Read the model definition and answer for the solid it produces. Units are mm, in the model's axes. A direction names the side the tool comes from. Give positions to 0.01 mm unless a question says otherwise; leave off trailing zeros. Loops run counter-clockwise (first coordinate to the right, second up) from the corner with the lowest first, then second, coordinate; pieces in that order, holes last. Notation, with made-up numbers: (73.25, -5) - (108.25, -5) arc R15 cw to (108.25, 23) - close; hole circle Ø9 at (88.25, 60). An arc over 180 degrees is marked (long way). Write each question's results on one line, items separated by ' | '. Start each with the question number.
Q1. Given pin 1 (2 mm diameter, centred on x = 74, z = -54, fed in from -Y); pin 2 (12 mm diameter, centred on x = 26.5, z = 53, fed in from +Y); pin 3 (6 mm diameter, centred on x = 40.5, y = -30.5, fed in from -Z) (3 decimals); pin 4 (11.5 mm diameter, centred on x = 39.4, y = 76.21, fed in from -Z) (3 decimals), each flat-ended and moving along its own axis, determine where each tip first touches the part or whether it passes through.
Q2. The part is cut by section B-B, the plane y = 39. Write down the section's boundary in (x, z) (3 decimals).
Q3. The part is cut by section C-C, the plane z = 22.5. Write down the section's boundary in (x, y).
Q4. Find the intervals of material crossed by line 1 (Z direction, x = 56.5, y = 29.5) (3 decimals); line 2 (Z direction, x = 36, y = 65.5) (3 decimals); line 3 (X direction, y = -33.5, z = -32), in increasing order. Write a range as from..to.
Q5. For faces 4 (the cylindrical face through (55.6, 91.8, 8)), 5 (the flat face through (39, -31, -47.665)), 6 (the flat face through (39, -3.551, -42)), 7 (the flat face through (84, -23.649, -24)), 8 (the flat face through (71.08, 41.4, -72.78)), determine the directions among +Z, -Z, +X, -X, +Y, -Y from which every point of the face is accessible in a straight line to the end or side of a thin tool.
Q6. The part is cut by section A-A, the plane x = 39.4. State how many separate pieces and enclosed holes the cut face has, plus the area to 3 significant figures.
Q7. Determine the mould class of faces 1 (the flat face through (40, 47, 6.965)), 2 (the cylindrical face through (36.36, 72.24, 7.95)), 3 (the cylindrical face through (39.952, -40.946, -46.239)) for opening direction Y: +Y half, -Y half, draft (parallel to the pull), parting line (faces both ways), or undercut.
```python
from build123d import *

# Parameters (mm, degrees)
BOSS_EXTRUDE1_DEPTH = 78.8
BOSS_EXTRUDE2_DEPTH = 2
FILLET2_R           = 10
BOSS_EXTRUDE3_DEPTH = 2
FILLET3_R           = 10
FILLET6_R           = 5
CUT_EXTRUDE1_REACH  = 193.572
SKETCH6_R           = 5
BOSS_EXTRUDE4_DEPTH = 10
CUT_EXTRUDE2_REACH  = 166.406
SKETCH10_W          = 52.85
SKETCH10_H          = 2
BOSS_EXTRUDE5_DEPTH = 2
SKETCH11_W          = 2
SKETCH11_H          = 52.85
BOSS_EXTRUDE6_DEPTH = 30.1
CUT_EXTRUDE3_DEPTH  = 2
FILLET9_R           = 5
FILLET11_R          = 2
SKETCH13_R          = 4.9
BOSS_EXTRUDE7_DEPTH = 10


with BuildPart() as part:
    # Sketch2 → Boss-Extrude1 (new body)
    with BuildSketch(Plane(origin=(0, 0, 0), x_dir=(0, 0, -1), z_dir=(1, 0, 0))):
        with BuildLine():
            Line((73.765, -25.649165393), (47.665, -25.649165393))
            Line((47.665, -25.649165393), (47.665, -42.449165393))
            Line((47.665, -42.449165393), (-58.695, -42.449165393))
            Line((-58.695, -42.449165393), (-73.765, -27.949165393))
            Line((-73.765, -27.949165393), (-73.765, 41.230834607))
            Line((-73.765, 41.230834607), (-6.965, 41.230834607))
            Line((-6.965, 41.230834607), (-6.965, 16.448577099))
            ThreePointArc((-6.965, 16.448577099), (-1.107135624, 2.306441476), (13.035, -3.551422901))
            Line((13.035, -3.551422901), (73.765, -3.551422901))
            Line((73.765, -3.551422901), (73.765, -25.649165393))
        make_face()
    extrude(amount=BOSS_EXTRUDE1_DEPTH)

    # Sketch4 → Boss-Extrude2 (add)
    with BuildSketch(Plane(origin=(0, 0, -73.765), x_dir=(-1, 0, 0), z_dir=(0, 0, -1))):
        Polygon((-78.8, -3.551422901), (0, -3.551422901), (-16.65, 93.408577099), (-62.15, 93.408577099), align=None)
    extrude(amount=-BOSS_EXTRUDE2_DEPTH)

    # Fillet2
    fillet2_edges = [part.edges().sort_by_distance(p)[0] for p in [
        (62.15, 93.408577099, -72.765),
        (16.65, 93.408577099, -72.765),
    ]]
    fillet(fillet2_edges, radius=FILLET2_R)

    # Sketch5 → Boss-Extrude3 (add)
    with BuildSketch(Plane(origin=(0, 0, 6.965), x_dir=(-1, 0, 0), z_dir=(0, 0, -1))):
        Polygon((-78.8, 41.230834607), (0, 41.230834607), (-22, 93.408577099), (-56.8, 93.408577099), align=None)
    extrude(amount=-BOSS_EXTRUDE3_DEPTH)

    # Fillet3
    fillet3_edges = [part.edges().sort_by_distance(p)[0] for p in [
        (56.8, 93.408577099, 7.965),
        (22, 93.408577099, 7.965),
    ]]
    fillet(fillet3_edges, radius=FILLET3_R)

    # Fillet6
    fillet6_edges = [part.edges().sort_by_distance(p)[0] for p in [
        (39.4, 41.230834607, 73.765),
        (39.4, -25.649165393, -73.765),
        (39.4, -42.449165393, -47.665),
        (39.4, -42.449165393, 58.695),
        (39.4, -27.949165393, 73.765),
    ]]
    fillet(fillet6_edges, radius=FILLET6_R)

    # Cut-Extrude1: up to this face of the body (flat: up to its plane)
    cut_extrude1_end = Plane(part.part.faces().sort_by_distance((39.4, 63.802944074, 8.965))[0])
    # Sketch6 → Cut-Extrude1 (cut, up to the picked face)
    with BuildSketch(Plane(origin=(0, 0, -73.765), x_dir=(-1, 0, 0), z_dir=(0, 0, -1)), mode=Mode.PRIVATE) as cut_extrude1_sk1:
        with Locations(Location((-39.4, 76.208577099, 0), (0, 0, 90))):
            Circle(SKETCH6_R)
    cut_extrude1_tool1 = split(extrude(cut_extrude1_sk1.sketch, amount=-CUT_EXTRUDE1_REACH, mode=Mode.PRIVATE), bisect_by=cut_extrude1_end, keep=Keep.BOTH, mode=Mode.PRIVATE)
    add(cut_extrude1_tool1.solids().sort_by(Axis((39.4, 76.208577, -73.765), (0, 0, 1)))[0], mode=Mode.SUBTRACT)

    # Sketch7 → Boss-Extrude4 (add)
    with BuildSketch(Plane(origin=(78.8, 0, 0), x_dir=(0, 0, -1), z_dir=(1, 0, 0))):
        Polygon((54.225, -25.649165393), (47.665, -25.649165393), (-4.955, -25.649165393), (-4.955, -23.649165393), (54.225, -23.649165393), align=None)
    extrude(amount=BOSS_EXTRUDE4_DEPTH)

    # Sketch9 → Cut-Extrude2 (cut, up to next)
    with BuildSketch(Plane(origin=(0, -23.649165393, 0), x_dir=(1, 0, 0), z_dir=(0, 1, 0)), mode=Mode.PRIVATE) as cut_extrude2_sk1:
        Polygon((88.8, 51.06), (78.8, 54.225), (88.8, 54.225), align=None)
    cut_extrude2_tool1 = extrude(cut_extrude2_sk1.sketch, amount=-CUT_EXTRUDE2_REACH, mode=Mode.PRIVATE) & part.part
    # Sketch9 → Cut-Extrude2 (cut, up to next)
    with BuildSketch(Plane(origin=(0, -23.649165393, 0), x_dir=(1, 0, 0), z_dir=(0, 1, 0)), mode=Mode.PRIVATE) as cut_extrude2_sk2:
        Polygon((88.8, -1.79), (78.8, -4.955), (88.8, -4.955), align=None)
    cut_extrude2_tool2 = extrude(cut_extrude2_sk2.sketch, amount=-CUT_EXTRUDE2_REACH, mode=Mode.PRIVATE) & part.part
    add(cut_extrude2_tool1.solids().sort_by_distance((85.466667, -23.649165, -53.17))[0], mode=Mode.SUBTRACT)
    add(cut_extrude2_tool2.solids().sort_by_distance((85.466667, -23.649165, 3.9))[0], mode=Mode.SUBTRACT)

    # Sketch10 → Boss-Extrude5 (add)
    with BuildSketch(Plane(origin=(88.8, 0, 0), x_dir=(0, 0, -1), z_dir=(1, 0, 0))):
        with Locations((24.635, -24.649165393)):
            Rectangle(SKETCH10_W, SKETCH10_H)
    extrude(amount=BOSS_EXTRUDE5_DEPTH)

    # Sketch11 → Boss-Extrude6 (add)
    with BuildSketch(Plane.XZ.offset(25.649165393)):
        with Locations((89.8, -24.635)):
            Rectangle(SKETCH11_W, SKETCH11_H)
    extrude(amount=BOSS_EXTRUDE6_DEPTH)

    # Sketch12 → Cut-Extrude3 (cut)
    with BuildSketch(Plane(origin=(90.8, 0, 0), x_dir=(0, 0, -1), z_dir=(1, 0, 0))):
        Polygon((9.82, -55.749165393), (-1.79, -23.649165393), (-1.79, -55.749165393), align=None)
        Polygon((39.45, -55.749165393), (51.06, -23.649165393), (51.06, -55.749165393), align=None)
    extrude(amount=-CUT_EXTRUDE3_DEPTH, mode=Mode.SUBTRACT)

    # Fillet9
    fillet9_edges = [part.edges().sort_by_distance(p)[0] for p in [
        (89.8, -55.749165393, -9.82),
        (89.8, -55.749165393, -39.45),
    ]]
    fillet(fillet9_edges, radius=FILLET9_R)

    # Fillet11
    fillet11_edges = [part.edges().sort_by_distance(p)[0] for p in [
        (90.8, -23.649165393, -24.635),
    ]]
    fillet(fillet11_edges, radius=FILLET11_R)

    # Sketch13 → Boss-Extrude7 (add)
    with BuildSketch(Plane.XZ.offset(42.449165393)):
        with Locations(Location((39.4, -24.265, 0), (0, 0, 90))):
            Circle(SKETCH13_R)
    extrude(amount=BOSS_EXTRUDE7_DEPTH)


solid = part.part
```
Check sheet entries:
1) pin 1: stops at y = -25.65 | pin 2: stops at y = 41.23 | pin 3: stops at z = -47.665 | pin 4: stops at z = -73.765
2) outline: (0, 6.965) - (78.8, 6.965) - (78.8, 72.928) - (0, 72.928) - close; (7.307, -73.765) - (71.493, -73.765) - (71.493, -71.765) - (7.307, -71.765) - close
3) outline: (0, -42.45) - (78.8, -42.45) - (78.8, 41.23) - (0, 41.23) - close
4) line 1: z = -73.765..-71.765, 6.965..73.765 | line 2: z = -73.765..-71.765, 6.965..8.965 | line 3: x = 0..78.8, 88.8..90.8
5) face 4: +Z, +X, +Y | face 5: -Z, -X, -Y | face 6: +X, -X, +Y | face 7: +Z, -Z, +X, +Y | face 8: -Z, +X, +Y
6) separate pieces: 3 | enclosed holes: 0 | area: 8,610 mm^2
7) face 1: draft | face 2: undercut | face 3: -Y half
